```python
from build123d import *

# Parameters (mm, degrees)
SKETCH_1_W          = 23.5
SKETCH_1_H          = 37.5
EXTRUDE_1_DEPTH     = 1.5
FILLET_1_R          = 1.5
EXTRUDE_2_DEPTH     = 5
SKETCH_3_W          = 2
SKETCH_3_H          = 4
CUT_EXTRUDE_1_DEPTH = 11
SKETCH_4_W          = 2
SKETCH_4_H          = 4
CUT_EXTRUDE_2_DEPTH = 12
SKETCH_5_W          = 2
SKETCH_5_H          = 3
CUT_EXTRUDE_3_DEPTH = 12
FILLET_2_R          = 1
SKETCH_6_R          = 0.9
CUT_EXTRUDE_4_DEPTH = 12
SKETCH_7_W          = 10
SKETCH_7_H          = 10
CUT_EXTRUDE_5_DEPTH = 12
SKETCH_8_W          = 5.533466027
SKETCH_8_H          = 3.21445342
CUT_EXTRUDE_6_DEPTH = 10
FILLET_3_R          = 1.5


with BuildPart() as part:
    # 草图1 → 凸台-拉伸1 (new body)
    with BuildSketch(Plane(origin=(0, 0, 0), x_dir=(1, 0, 0), z_dir=(0, 1, 0))):
        Rectangle(SKETCH_1_W, SKETCH_1_H)
    extrude(amount=EXTRUDE_1_DEPTH)

    # 圆角1
    fillet_1_edges = [part.edges().sort_by_distance(p)[0] for p in [
        (-11.75, 0.75, -18.75),
        (11.75, 0.75, -18.75),
        (11.75, 0.75, 18.75),
        (-11.75, 0.75, 18.75),
    ]]
    fillet(fillet_1_edges, radius=FILLET_1_R)

    # 草图2 → 凸台-拉伸2 (add)
    with BuildSketch(Plane(origin=(0, 1.5, 0), x_dir=(1, 0, 0), z_dir=(0, 1, 0))):
        Polygon((-8.792128206, -17.15), (10.15, -17.15), (10.15, 8), (8.15, 8), (8.15, -15.15), (-8.15, -15.15), (-8.15, 8), (-10.15, 8), (-10.15, -17.15), align=None)
    extrude(amount=EXTRUDE_2_DEPTH)

    # 草图3 → 切除-拉伸1 (cut)
    with BuildSketch(Plane.ZY.offset(10.15)):
        with Locations((16.15, 4.5)):
            Rectangle(SKETCH_3_W, SKETCH_3_H)
    extrude(amount=-CUT_EXTRUDE_1_DEPTH, mode=Mode.SUBTRACT)

    # 草图4 → 切除-拉伸2 (cut)
    with BuildSketch(Plane.XY.offset(15.15)):
        with Locations((-9.15, 4.5)):
            Rectangle(SKETCH_4_W, SKETCH_4_H)
    extrude(amount=-CUT_EXTRUDE_2_DEPTH, mode=Mode.SUBTRACT)

    # 草图5 → 切除-拉伸3 (cut)
    with BuildSketch(Plane.ZY.offset(-0.85)):
        with Locations((16.15, 5)):
            Rectangle(SKETCH_5_W, SKETCH_5_H)
    extrude(amount=-CUT_EXTRUDE_3_DEPTH, mode=Mode.SUBTRACT)

    # 圆角2
    fillet_2_edges = [part.edges().sort_by_distance(p)[0] for p in [
        (0, 1.5, 15.15),
        (-8.15, 1.5, 3.575),
        (8.15, 1.5, 3.575),
    ]]
    fillet(fillet_2_edges, radius=FILLET_2_R - 0.0001)  # a hair under: the kernel refuses the full size

    # 草图6 → 切除-拉伸4 (cut)
    with BuildSketch(Plane(origin=(10.15, 0, 0), x_dir=(0, 0, -1), z_dir=(1, 0, 0))):
        with Locations((0, 4.5)):
            Circle(SKETCH_6_R)
    extrude(amount=-CUT_EXTRUDE_4_DEPTH, mode=Mode.SUBTRACT)

    # 草图7 → 切除-拉伸5 (cut)
    with BuildSketch(Plane.XZ):
        with Locations((5.25, -12.25)):
            Rectangle(SKETCH_7_W, SKETCH_7_H)
    extrude(amount=-CUT_EXTRUDE_5_DEPTH, mode=Mode.SUBTRACT)

    # 草图8 → 切除-拉伸6 (cut)
    with BuildSketch(Plane(origin=(10.15, 0, 0), x_dir=(0, 0, -1), z_dir=(1, 0, 0))):
        with Locations((4.483266987, 4.89277329)):
            Rectangle(SKETCH_8_W, SKETCH_8_H)
    extrude(amount=-CUT_EXTRUDE_6_DEPTH, mode=Mode.SUBTRACT)

    # 圆角3
    fillet_3_edges = [part.edges().sort_by_distance(p)[0] for p in [
        (9.15, 6.5, -1.716533973),
    ]]
    fillet(fillet_3_edges, radius=FILLET_3_R)


solid = part.part
```
Geometry: final body of the model. Coordinates: model frame, mm. A direction names the side the tool comes from. Round coordinates to 2 decimals unless told otherwise and drop trailing zeros. Order: outer loops, then holes, each group sorted by start corner. A loop starts at its lowest first (then second) coordinate and runs counter-clockwise, first axis right, second up. Notation, with made-up numbers: (16, -18) -> (47, -18) arc R13 ccw to (47, -4) -> close; hole circle Ø9 at (68, -18.75). An arc over 180 degrees is marked (long way). Use one line per item in the form item = value. Start each with the question number.
1. Cut plane A-A (y = 4.5). Return the cut outline in (x, z), then the cut area to 3 significant figures.
2. Reachability of faces 1 (the face through (9, 4, -1.717)), 2 (the face through (9, 5, 15.15)), 3 (the face through (10.15, 3, 5)) from +Z, -Z, +X, -X, +Y, -Y: full face, straight path, thin tool, end or side. Return the list, or none.
3. Line query: probe 1 along Y at (x, z) = (9.45, 0); probe 2 along Z at (x, y) = (2.25, 0.75); probe 3 along X at (y, z) = (3.5, 2). Output: solid intervals per line, ascending.
4. Cut plane B-B (x = 4.5). Return the cut outline in (y, z).
5. Draft query along X for faces 4 (the face through (-11.32, 0.76, -18.3)), 5 (the face through (0, 1, 18.75)), 6 (the face through (-8.15, 4, -1)), 7 (the face through (7.849, 1.785, 4.107)). Return one class per face: pulls with the +X half, pulls with the -X half, needs draft (parallel to the pull), parting line crosses it, or undercut.
6. Cut plane C-C (z = -6). Return the cut outline in (x, y), then the cut area to 3 significant figures.
7. Pin query (flat end, axial travel): pin 1 Ø0.9 at (x, y) = (8.5, 4.5) entering from -Z; pin 2 Ø1.1 at (x, y) = (4, 3) entering from -Z; pin 3 Ø12 at (x, z) = (-1, 1) entering from +Y. Return the tip coordinate at first contact, or that it passes through.
Solution:
q1.outline = (-10.15, -8) -> (-8.15, -8) -> (-8.15, 3.15) -> (-10.15, 3.15) -> close; (8.15, -1.72) -> (10.15, -1.72) -> (10.15, -0.9) -> (8.15, -0.9) -> close; (8.15, 0.9) -> (10.15, 0.9) -> (10.15, 15.15) -> (8.15, 15.15) -> close
q1.area = 52.4 mm^2
q2.face_1 = -Z, +X, +Y
q2.face_2 = +Z, +X, -X, +Y
q2.face_3 = +Z, -Z, +X, +Y
q3.probe_1 = 0 to 3.6, 5.4 to 6.5
q3.probe_2 = -18.75 to -17.25, -7.25 to 18.75
q3.probe_3 = -10.15 to -8.15, 8.15 to 10.15
q4.outline = (0, -18.75) -> (1.5, -18.75) -> (1.5, -17.25) -> (0, -17.25) -> close; (0, -7.25) -> (1.5, -7.25) -> (1.5, 14.15) arc R1 cw to (2.5, 15.15) -> (3.5, 15.15) -> (3.5, 17.15) -> (1.5, 17.15) -> (1.5, 18.75) -> (0, 18.75) -> close
q5.face_4 = pulls with the -X half
q5.face_5 = needs draft
q5.face_6 = undercut
q5.face_7 = undercut
q6.outline = (-11.75, 0) -> (11.75, 0) -> (11.75, 1.5) -> (10.15, 1.5) -> (10.15, 3.29) -> (8.15, 3.29) -> (8.15, 2.5) arc R1 cw to (7.15, 1.5) -> (-7.15, 1.5) arc R1 cw to (-8.15, 2.5) -> (-8.15, 6.5) -> (-10.15, 6.5) -> (-10.15, 1.5) -> (-11.75, 1.5) -> close
q6.area = 49.3 mm^2
q7.pin_1 = -1.72
q7.pin_2 = 15.15
q7.pin_3 = 1.5
